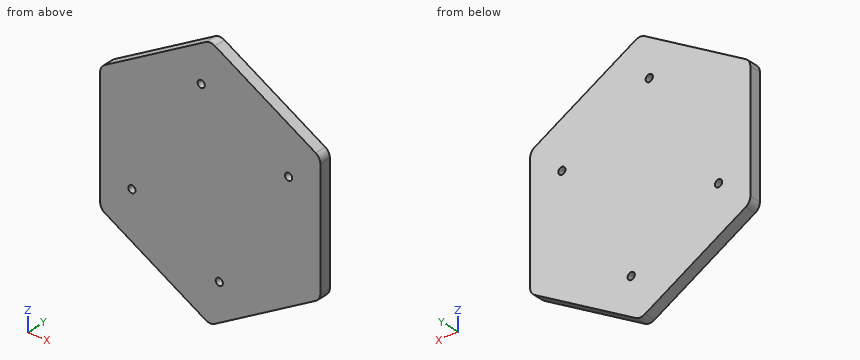
Autodesk Inventor part; units mm, degrees
ref_plane "YZ Plane" through (0, 0, 0) normal (1, 0, 0) x (0, 1, 0)
ref_plane "XZ Plane" through (0, 0, 0) normal (0, 1, 0) x (-1, 0, 0)
ref_plane "XY Plane" through (0, 0, 0) normal (0, 0, 1) x (1, 0, 0)
sketch "Sketch1" plane through (0, 0, 0) normal (0, 1, 0) x (-1, 0, 0)
  line L0 (-47.5136, -27.432) -> (-47.5136, 27.432)
  line L1 (-47.5136, 27.432) -> (0, 54.864)
  line L2 (0, 54.864) -> (47.5136, 27.432)
  line L3 (47.5136, 27.432) -> (47.5136, -27.432)
  line L4 (47.5136, -27.432) -> (0, -54.864)
  line L5 (0, -54.864) -> (-47.5136, -27.432)
  line L6 (0, 54.864) -> (47.5136, 27.432)
  line L7 (47.5136, 27.432) -> (47.5136, -27.432)
  line L8 (47.5136, -27.432) -> (0, -54.864)
  line L9 (0, -54.864) -> (-47.5136, -27.432)
  line L10 (-47.5136, -27.432) -> (-47.5136, 27.432)
  line L11 (-47.5136, 27.432) -> (0, 54.864)
  line L12 (0, 54.805) -> (-47.4625, 27.4025)
  line L13 (-47.4625, 27.4025) -> (-47.4625, -27.4025)
  line L14 (-47.4625, -27.4025) -> (0, -54.805)
  line L15 (-47.4625, 27.4025) -> (0, 54.805)
  line L16 (0, 54.805) -> (47.4625, 27.4025)
  line L17 (47.4625, 27.4025) -> (47.4625, -27.4025)
  line L18 (47.4625, -27.4025) -> (0, -54.805)
  line L19 (0, -54.805) -> (-47.4625, -27.4025)
  line L20 (-47.4625, -27.4025) -> (-47.4625, 27.4025)
  circle A0 centre (-33.775, 15) radius 1.55
  circle A1 centre (-3.8971, -36.75) radius 1.55
  circle A2 centre (33.775, -15) radius 1.55
  circle A3 centre (3.8971, 36.75) radius 1.55
  line L21 (-33.775, 19.5) -> (0, 39) construction
  line L22 (0, 39) -> (33.775, 19.5) construction
  line L23 (33.775, 19.5) -> (33.775, -19.5) construction
  line L24 (33.775, -19.5) -> (0, -39) construction
  line L25 (0, -39) -> (-33.775, -19.5) construction
  line L26 (-33.775, -19.5) -> (-33.775, 19.5) construction
  line L27 (-44.5136, -25.6999) -> (-44.5136, 25.6999)
  line L28 (-44.5136, 25.6999) -> (0, 51.3999)
  line L29 (0, 51.3999) -> (44.5136, 25.6999)
  line L30 (44.5136, 25.6999) -> (44.5136, -25.6999)
  line L31 (0, -51.3999) -> (-44.5136, -25.6999)
  line L32 (47.5136, -27.432) -> (47.5136, 27.432)
  line L33 (47.5136, 27.432) -> (0, 54.864)
  line L34 (0, 54.864) -> (-47.5136, 27.432)
  line L35 (-47.5136, 27.432) -> (-47.5136, -27.432)
  line L36 (-47.5136, -27.432) -> (0, -54.864)
  line L37 (0, -54.864) -> (47.5136, -27.432)
  line L38 (44.5136, 25.6999) -> (44.5136, -25.6999)
  line L39 (29.2636, 11) -> (29.2636, -11)
  line L40 (44.5136, -11) -> (44.5136, 11)
  line L41 (44.5136, 0) -> (46.3422, 0) construction
  line L42 (0, -33.7907) -> (-29.2636, -16.8954) construction
  line L43 (-29.2636, -16.8954) -> (-29.2636, 16.8954) construction
  line L44 (-29.2636, 16.8954) -> (-16.4566, 24.2895) construction
  line L45 (0, 33.7907) -> (29.2636, 16.8954) construction
  line L46 (29.2636, 16.8954) -> (29.2636, -16.8954) construction
  line L47 (29.2636, -16.8954) -> (16.4566, -24.2895) construction
  line L48 (0, -51.3999) -> (-44.5136, -25.6999) construction
  line L49 (20.432, -39.6035) -> (0, -51.3999) construction
  line L50 (44.5136, -25.6999) -> (24.0816, -37.4964) construction
  line L51 (44.5136, 25.6999) -> (44.5136, -25.6999) construction
  line L52 (0, 51.3999) -> (44.5136, 25.6999) construction
  line L53 (-20.432, 39.6035) -> (0, 51.3999) construction
  line L54 (-44.5136, 25.6999) -> (-24.0816, 37.4964) construction
  line L55 (-44.5136, -25.6999) -> (-44.5136, 25.6999) construction
  line L56 (29.2636, 16.8954) -> (0, 33.7907)
  line L57 (31.7831, 33.0499) -> (12.7305, 44.0499)
  line L58 (22.2568, 38.5499) -> (22.6365, 39.2076)
  line L59 (0, 51.3999) -> (44.5136, 25.6999)
  line L60 (0, 33.7907) -> (29.2636, 16.8954)
  line L61 (0, 0) -> (0, -5.712) construction
  line L62 (0, 0) -> (4.8403, -2.7945) construction
  line L63 (29.2636, 16.8954) -> (29.2636, -16.8954) construction
  line L64 (-44.5136, -11) -> (-44.5136, 11)
  line L65 (-22.2568, -38.5499) -> (-22.6365, -39.2076)
  line L66 (-12.7305, -44.0499) -> (-31.7831, -33.0499)
  line L67 (-24.1581, -19.843) -> (-5.1055, -30.843)
  line L68 (0, -54.864) -> (47.5136, -27.432) construction
  line L69 (23.7568, -41.148) -> (25.1641, -43.5855) construction
  line L70 (29.2636, -16.8954) -> (0, -33.7907)
  line L71 (0, 0) -> (6.6102, 3.8164) construction
  line L72 (0, 51.3999) -> (-44.5136, 25.6999)
  line L73 (0, 33.7907) -> (-29.2636, 16.8954) construction
  line L74 (-24.1581, 19.843) -> (-31.7831, 33.0499)
  line L75 (-31.7831, 33.0499) -> (-12.7305, 44.0499)
  line L76 (5.1055, -30.843) -> (24.1581, -19.843)
  line L77 (0, -33.7907) -> (29.2636, -16.8954)
  line L78 (41.3094, 27.5499) -> (29.4425, 34.4013)
  line L79 (31.7831, 33.0499) -> (12.7305, 44.0499)
  line L80 (-12.7305, 44.0499) -> (-31.7831, 33.0499)
  line L81 (-31.7831, 33.0499) -> (-24.1581, 19.843)
  line L82 (-5.1055, -30.843) -> (-24.1581, -19.843)
  line L83 (0, -33.7907) -> (-29.2636, -16.8954)
  line L84 (-31.7831, -33.0499) -> (-12.7305, -44.0499)
  line L85 (12.807, -26.3966) -> (0, -33.7907)
  line L86 (-12.807, 26.3966) -> (0, 33.7907)
  point P0 (-44.5136, 0)
  point P1 (-44.5136, 0)
  dimension "d0" = 54.864
  dimension "d1" = 0
  dimension "d3" = 39
  dimension "d6" = 4.5
  dimension "d7" = 4.5
  dimension "d11" = 4.5
  dimension "d15" = 4.5
extrude "Extrusion2" add sketch "Sketch1" along normal blind 5 contours L16 L17 L18 L14 L13 L12
fillet "Fillet1" radius 4 6 edges at (47.4625, 2.5, 27.4025) (0, 2.5, 54.805) (-47.4625, 2.5, 27.4025) (-47.4625, 2.5, -27.4025) (0, 2.5, -54.805) (47.4625, 2.5, -27.4025)
equation "\"d6\" = d4"
equation "\"d7\" = d5"
equation "\"d11\" = d4"
equation "\"d15\" = d9"
equation "\"d5\" = d4"
equation "\"d9\" = d4"
properties part number "tapa"
The model under review builds one solid part; all positions refer to its coordinate system, in mm. Give positions to 0.01 mm unless a question says otherwise; leave off trailing zeros. Order: outer loops, then holes, each group sorted by start corner. A loop starts at its lowest first (then second) coordinate and runs counter-clockwise, first axis right, second up. Notation, with made-up numbers: M 46.5,81 L 64.5,81 A14 ccw 64.5,89 Z; hole C -21,10.25 d3. An arc over 180 degrees is marked long. One line per question, with ' | ' between items. Start each with the question number.
1) Clearance check with a flat-ended pin moving along its axis: P1, Ø1, axis at y = 4, z = 33.5, coming from the +X side. State where the tip first meets the part, or that it passes through.
2) Consider section A-A, the plane z = -15. Give the boundary of the cut face in (x, y) (1 decimal), then the cut area to 3 significant figures.
3) Consider section D-D, the plane x = -31. Give the boundary of the cut face in (y, z), then the cut area to 3 significant figures.
4) Consider section C-C, the plane z = 36.75. Give the boundary of the cut face in (x, y), then the cut area to 3 significant figures.
5) Wall thickness on L1, parallel to X at y = 3.95, z = -25.5; L2, parallel to Z at x = 43, y = 4.5; L3, parallel to Z at x = -14, y = 4.5: over which ranges is each line inside the solid? List them lowest first. Write a range as from..to.
6) Consider section B-B, the plane y = 2.1. State how many separate pieces and enclosed holes the cut face has, then the cut area to 3 significant figures.
Found:
1) P1: stops at x = 37.77
2) outline: M -47.5,0 L -35.3,0 L -35.3,5 L -47.5,5 Z; M -32.2,0 L 47.5,0 L 47.5,5 L -32.2,5 Z | area: 459 mm²
3) outline: M 0,-36.91 L 5,-36.91 L 5,36.91 L 0,36.91 Z | area: 369 mm²
4) outline: M -31.27,0 L -5.45,0 L -5.45,5 L -31.27,5 Z; M -2.35,0 L 31.27,0 L 31.27,5 L -2.35,5 Z | area: 297 mm²
5) L1: x = -47.44..47.44 | L2: z = -29.98..29.98 | L3: z = -46.72..46.72
6) separate pieces: 1 | enclosed holes: 4 | area: 7,770 mm²
